Drawing for the job (mm, zero at the part's lowest x, y, z). A direction names the side the tool comes from. Give positions to 0.01 mm unless a question says otherwise; leave off trailing zeros. Order: outer loops, then holes, each group sorted by start corner. A loop starts at its lowest first (then second) coordinate and runs counter-clockwise, first axis right, second up. Notation, with made-up numbers: (2, 74.5) - (38, 74.5) arc R9 cw to (38, 83.5) - close; hole circle Ø9 at (-0.5, -9.75). An arc over 180 degrees is marked (long way). One line per item, written item: value.
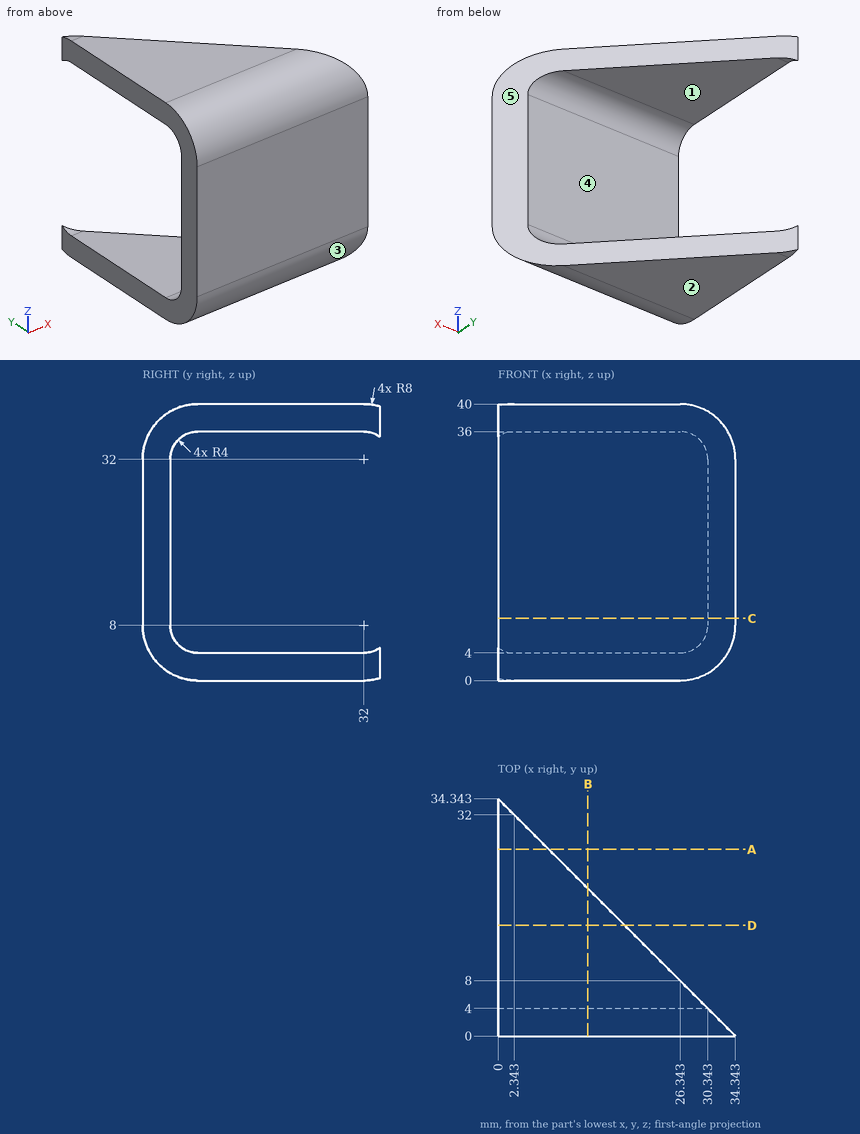
1) Cut at A-A, the plane y = 27. Give the cut face in (x, z).
Outcome:
outline: (0, 0) - (7.34, 0) - (7.34, 4) - (0, 4) - close; (0, 36) - (7.34, 36) - (7.34, 40) - (0, 40) - close
2) Cut at D-D, the plane y = 16. Give the cut face in (x, z), then the cut area to 3 significant figures.
Outcome:
outline: (0, 0) - (18.34, 0) - (18.34, 4) - (0, 4) - close; (0, 36) - (18.34, 36) - (18.34, 40) - (0, 40) - close
area: 147 mm^2
3) Cut at B-B, the plane x = 13. Give the cut face in (y, z), then the cut area to 3 significant figures.
Outcome:
outline: (0, 8) arc R8 ccw to (8, 0) - (21.34, 0) - (21.34, 4) - (8, 4) arc R4 cw to (4, 8) - (4, 32) arc R4 cw to (8, 36) - (21.34, 36) - (21.34, 40) - (8, 40) arc R8 ccw to (0, 32) - close
area: 278 mm^2
4) Pin check, flat tips, straight feed: pin 1 (1 mm diameter, centred on x = 21, z = 22, fed in from +Y); pin 2 (1.5 mm diameter, centred on x = 10, y = 28, fed in from +Z); pin 3 (1.5 mm diameter, centred on y = 4, z = 8, fed in from +X). Stop position of each tip, or through.
Outcome:
pin 1: stops at y = 4
pin 2: passes through
pin 3: stops at x = 31.09
5) Cut at C-C, the plane z = 9. Give the cut face in (x, y), then the cut area to 3 significant figures.
Outcome:
outline: (0, 0) - (34.34, 0) - (30.34, 4) - (0, 4) - close
area: 129 mm^2
6) Mould opens along Z. For the marked faces 3, 4 and 5 say: released by +Z, released by -Z, zero draft, split by the parting line, or undercut.
Outcome:
face 3: released by -Z
face 4: undercut
face 5: zero draft
7) Which spindle directions (+Z, -Z, +X, -X, +Y, -Y) get a long thin tool onto all of the face, cutting with end or side? Do the marked faces 1 and 2. Say none if no direction does.
Outcome:
face 1: +X, -X
face 2: -Z, +X, -X, +Y, -Y
8) Drill centre lines: line 1 along Z through (x, y) = (14.5, 13.5); line 2 along Y through (x, z) = (11, 11); line 3 along Z through (x, y) = (25.5, 7). Where is each one in solid material? Low to high. Write a range as from..to.
Outcome:
line 1: z = 0..4, 36..40
line 2: y = 0..4
line 3: z = 0.06..4.13, 35.87..39.94
